from build123d import *

# Parameters (mm, degrees)
BOSS_EXTRUDE1_DEPTH = 7.5
SKETCH2_R           = 3
CUT_EXTRUDE1_DEPTH  = 15
SKETCH3_R           = 3
CUT_EXTRUDE2_DEPTH  = 55.371407927
FILLET1_R           = 6


with BuildPart() as part:
    # Sketch1 → Boss-Extrude1 (new, symmetric)
    with BuildSketch(Plane(origin=(0, 0, 0), x_dir=(0, 0, -1), z_dir=(1, 0, 0))):
        Polygon((0, 0), (-10, 0), (-10, -50), (-8, -50), (-8, -5), (8, -5), (8, -50), (10, -50), (10, 0), align=None)
    extrude(amount=BOSS_EXTRUDE1_DEPTH, both=True)

    # Sketch2 → Cut-Extrude1 (cut)
    with BuildSketch(Plane(origin=(0, 0, 0), x_dir=(1, 0, 0), z_dir=(0, 1, 0))):
        with Locations(Location((0, 0, 0), (0, 0, 270))):
            Circle(SKETCH2_R)
    extrude(amount=-CUT_EXTRUDE1_DEPTH, mode=Mode.SUBTRACT)

    # Sketch3 → Cut-Extrude2 (cut, through all)
    with BuildSketch(Plane.XY.offset(10)):
        with Locations((0, -42)):
            Circle(SKETCH3_R)
    extrude(amount=-CUT_EXTRUDE2_DEPTH, mode=Mode.SUBTRACT)

    # Fillet1
    fillet1_edges = [part.edges().sort_by_distance(p)[0] for p in [
        (-7.5, -50, 9),
        (0, 0, -10),
        (0, 0, 10),
        (7.5, -50, 9),
        (7.5, -50, -9),
        (-7.5, -50, -9),
    ]]
    fillet(fillet1_edges, radius=FILLET1_R)


solid = part.part
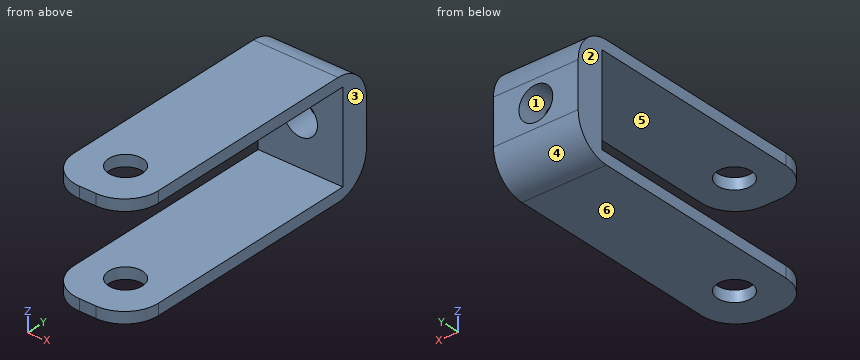
Check sheet for the modelled part. Datum: model origin and axes. Units: mm. Face numbers are marked on the shaded views. A direction names the side the tool comes from. Coordinates: 2 decimals unless noted, no trailing zeros. Loops run counter-clockwise (first coordinate to the right, second up) from the corner with the lowest first, then second, coordinate; pieces in that order, holes last. Notation, with made-up numbers: (-2.5, -13) -> (37.5, -13) arc R17 cw to (37.5, 9) -> close; hole circle Ø10 at (32, 24). An arc over 180 degrees is marked (long way). Answer in a Markdown table with one row per item.
1. Material ranges on line 1 along Z through (x, y) = (3.5, -36); line 2 along X through (y, z) = (-2.9, 0); line 3 along Y through (x, z) = (2, 2.5), recorded low to high. Write a range as [from, to].
Check values:
| item | result |
|---|---|
| line 1 | z = [-10, -8], [8, 10] |
| line 2 | x = [-7.5, -3], [3, 7.5] |
| line 3 | y = [-5, 0] |
2. Sectioned sample at A-A, the plane y = -42. Record the boundary of the cut face in (x, z).
Check values:
| item | result |
|---|---|
| outline | (-7.5, -10) -> (-3, -10) -> (-3, -8) -> (-7.5, -8) -> close; (-7.5, 8) -> (-3, 8) -> (-3, 10) -> (-7.5, 10) -> close; (3, -10) -> (7.5, -10) -> (7.5, -8) -> (3, -8) -> close; (3, 8) -> (7.5, 8) -> (7.5, 10) -> (3, 10) -> close |
3. Go/stop test with flat-tipped pins: pin 1 (12 mm diameter, centred on y = -13, z = -4, fed in from -X); pin 2 (3 mm diameter, centred on x = 0, z = -4, fed in from -Y); pin 3 (8 mm diameter, centred on y = -44, z = 2.5, fed in from -X). Record where each tip stops, or that it passes through.
Check values:
| item | result |
|---|---|
| pin 1 | stops at x = -7.5 |
| pin 2 | stops at y = -5 |
| pin 3 | passes through |
4. Sectioned sample at D-D, the plane z = 0. Record the boundary of the cut face in (x, y).
Check values:
| item | result |
|---|---|
| outline | (-7.5, -5) -> (-3, -5) -> (-3, 0) -> (-7.5, 0) -> close; (3, -5) -> (7.5, -5) -> (7.5, 0) -> (3, 0) -> close |
5. Sectioned sample at C-C, the plane x = 0. Record the boundary of the cut face in (y, z).
Check values:
| item | result |
|---|---|
| outline | (-50, -10) -> (-45, -10) -> (-45, -8) -> (-50, -8) -> close; (-50, 8) -> (-45, 8) -> (-45, 10) -> (-50, 10) -> close; (-39, -10) -> (-6, -10) arc R6 ccw to (0, -4) -> (0, -3) -> (-5, -3) -> (-5, -8) -> (-39, -8) -> close; (-39, 8) -> (-5, 8) -> (-5, 3) -> (0, 3) -> (0, 4) arc R6 ccw to (-6, 10) -> (-39, 10) -> close |
6. Sectioned sample at B-B, the plane y = -15.5. Record the boundary of the cut face in (x, z), then the cut area to 3 significant figures.
Check values:
| item | result |
|---|---|
| outline | (-7.5, -10) -> (7.5, -10) -> (7.5, -8) -> (-7.5, -8) -> close; (-7.5, 8) -> (7.5, 8) -> (7.5, 10) -> (-7.5, 10) -> close |
| area | 60.0 mm2 |
7. Access from +Z, -Z, +X, -X, +Y, -Y to the whole of each face (thin tool, end or side, straight path). Record for the marked faces 5 and 6.
Check values:
| item | result |
|---|---|
| face 5 | +X, -X, -Y |
| face 6 | -Z, +X, -X, +Y, -Y |
8. Release check for a two-part mould opening along X. For the marked faces 1, 2, 3 and 4 record: released by +X, released by -X, zero draft, split by the parting line, or undercut.
Check values:
| item | result |
|---|---|
| face 1 | undercut |
| face 2 | released by -X |
| face 3 | released by +X |
| face 4 | zero draft |
